Could you check a few things on this model? Use its own coordinates, in mm. A direction names the side the tool comes from. Give positions to 0.01 mm unless a question says otherwise; leave off trailing zeros. Loops run counter-clockwise (first coordinate to the right, second up) from the corner with the lowest first, then second, coordinate; pieces in that order, holes last. Notation, with made-up numbers: (44.25, -10) - (103.25, -10) arc R13 ccw to (103.25, 2) - close; hole circle Ø1 at (42.25, -5.75). An arc over 180 degrees is marked (long way). Answer in a Markdown table with one row per item. Add a question column.
```python
from build123d import *
from OCP.BRepFilletAPI import BRepFilletAPI_MakeChamfer

# Parameters (mm, degrees)
SKETCH1_W                     = 20
SKETCH1_H                     = 40.56076
BOSS_EXTRUDE1_DEPTH           = 8
SKETCH6_R                     = 1.4
CUT_EXTRUDE1_DEPTH            = 10
SKETCH8_R                     = 7.5
BOSS_EXTRUDE2_DEPTH           = 2.5
SKETCH9_R                     = 5.1
CUT_EXTRUDE3_DEPTH            = 4
SKETCH10_R                    = 3
CUT_EXTRUDE4_DEPTH            = 6.5
FILLET1_R                     = 2
CHAMFER1_SIZE2                = 2.5
CHAMFER1_SIZE                 = 1.8
SKETCH11_W                    = 8
SKETCH11_H                    = 7
CUT_EXTRUDE5_DEPTH            = 3.5
CHAMFER2_SIZE                 = 2.020725942
CHAMFER2_SIZE_2               = 3.5
FILLET2_R                     = 3
BODY_MOVE_COPY1_OUTLINE_W     = 2.1
BODY_MOVE_COPY1_OUTLINE_H     = 6.5
BODY_MOVE_COPY1_START         = -10
BODY_MOVE_COPY1_2_DEPTH       = 20
BODY_MOVE_COPY1_3_OUTLINE_R   = 1.4
BODY_MOVE_COPY1_3_DEPTH       = 4.176980959
BODY_MOVE_COPY1_4_OUTLINE_R   = 1.4
BODY_MOVE_COPY1_4_DEPTH       = 20
BODY_MOVE_COPY1_5_OUTLINE_R   = 1.4
BODY_MOVE_COPY1_5_DEPTH       = 10
BODY_MOVE_COPY1_6_OUTLINE_R   = 5.1
BODY_MOVE_COPY1_6_DEPTH       = 2.5
BODY_MOVE_COPY1_START_2       = -16
BODY_MOVE_COPY1_7_OUTLINE_R   = 3
BODY_MOVE_COPY1_7_DEPTH       = 8
BODY_MOVE_COPY1_8_OUTLINE_R   = 5.1
BODY_MOVE_COPY1_8_OUTLINE_R_2 = 3
BODY_MOVE_COPY1_8_DEPTH       = 1.5


with BuildPart() as part:
    # Sketch1 → Boss-Extrude1 (new body)
    with BuildSketch(Plane.XY):
        Rectangle(SKETCH1_W, SKETCH1_H)
    extrude(amount=-BOSS_EXTRUDE1_DEPTH)

    # Sketch6 → Cut-Extrude1 (cut)
    with BuildSketch(Plane(origin=(10, 0, 0), x_dir=(0, 0, -1), z_dir=(1, 0, 0))):
        with Locations(Location((3.3, -15.26519, 0), (0, 0, 180))):
            Circle(SKETCH6_R)
        with Locations((3.3, -5.26519)):
            Circle(SKETCH6_R)
        with Locations((3.3, 15.26519)):
            Circle(SKETCH6_R)
        with Locations(Location((3.3, 5.26519, 0), (0, 0, 180))):
            Circle(SKETCH6_R)
    extrude(amount=-CUT_EXTRUDE1_DEPTH, mode=Mode.SUBTRACT)

    # Sketch8 → Boss-Extrude2 (add)
    with BuildSketch(Plane.XY):
        Circle(SKETCH8_R)
    extrude(amount=BOSS_EXTRUDE2_DEPTH)

    # Sketch9 → Cut-Extrude3 (cut)
    with BuildSketch(Plane.XY.offset(2.5)):
        Circle(SKETCH9_R)
    extrude(amount=-CUT_EXTRUDE3_DEPTH, mode=Mode.SUBTRACT)

    # Sketch10 → Cut-Extrude4 (cut)
    with BuildSketch(Plane.XY.offset(-1.5)):
        Circle(SKETCH10_R)
    extrude(amount=-CUT_EXTRUDE4_DEPTH, mode=Mode.SUBTRACT)

    # Fillet1
    fillet1_edges = [part.edges().sort_by_distance(p)[0] for p in [
        (0, -20.28038, 0),
        (0, 20.28038, 0),
    ]]
    fillet(fillet1_edges, radius=FILLET1_R)

    # Chamfer1
    chamfer1_edges = [part.edges().sort_by_distance(p)[0] for p in [
        (-7.5, 0, 0),
    ]]
    chamfer1_side = [part.faces().sort_by_distance(p)[0] for p in [
        (-7.536, 0, 0),
    ]]
    chamfer(chamfer1_edges, length=CHAMFER1_SIZE - 0.0001, length2=CHAMFER1_SIZE2 - 0.0001, reference=chamfer1_side[0])  # a hair under: the kernel refuses the full size

    # Sketch11 → Cut-Extrude5 (cut)
    with BuildSketch(Plane.ZY.offset(10)):
        with Locations((-4, -10.26517)):
            Rectangle(SKETCH11_W, SKETCH11_H)
    extrude(amount=-CUT_EXTRUDE5_DEPTH, mode=Mode.SUBTRACT)

    # Chamfer2
    chamfer2_edges_1 = [part.edges().sort_by_distance(p)[0] for p in [
        (-10, -13.76517, -4),
    ]]
    chamfer2_side_1 = [part.faces().sort_by_distance(p)[0] for p in [
        (-10, -13.805584519, -4),
    ]]
    chamfer2_edges_2 = [part.edges().sort_by_distance(p)[0] for p in [
        (-10, -6.76517, -4),
    ]]
    chamfer2_side_2 = [part.faces().sort_by_distance(p)[0] for p in [
        (-9.959585481, -6.76517, -4),
    ]]
    chamfer2 = BRepFilletAPI_MakeChamfer(part.part.solid().wrapped)
    for e in chamfer2_edges_1:
        chamfer2.Add(CHAMFER2_SIZE - 0.0001, CHAMFER2_SIZE_2 - 0.0001, e.wrapped, chamfer2_side_1[0].wrapped)
    for e in chamfer2_edges_2:
        chamfer2.Add(CHAMFER2_SIZE_2 - 0.0001, CHAMFER2_SIZE - 0.0001, e.wrapped, chamfer2_side_2[0].wrapped)
    add(Compound.cast(chamfer2.Shape()), mode=Mode.REPLACE)  # a hair under: the kernel refuses the full size

    # Fillet2
    fillet2_edges = [part.edges().sort_by_distance(p)[0] for p in [
        (-10, -15.785795942, -4),
        (-10, -4.744544058, -4),
    ]]
    fillet(fillet2_edges, radius=FILLET2_R)

    # Body-Move/Copy1: read off the stored shape, not the designer's step
    # Body-Move/Copy1 outline → Body-Move/Copy1 (revolve)
    with BuildSketch(Plane.XZ):
        Polygon((7.5, -18.5), (9.3, -16), (5.1, -16), (5.1, -18.5), align=None)
        with Locations((4.05, -11.25)):
            Rectangle(BODY_MOVE_COPY1_OUTLINE_W, BODY_MOVE_COPY1_OUTLINE_H)
    revolve(axis=Axis((0, 0, 0), (0, 0, 1)))

    # Body-Move_Copy1 2 outline → Body-Move_Copy1 2 (cut)
    with BuildSketch(Plane.YZ.offset(BODY_MOVE_COPY1_START)):
        with BuildLine():
            Line((-20.28038, -8), (20.28038, -8))
            Line((20.28038, -8), (20.28038, -2))
            ThreePointArc((20.28038, -2), (19.694593562, -0.585786438), (18.28038, 0))
            Line((18.28038, 0), (-18.28038, 0))
            ThreePointArc((-18.28038, 0), (-19.694593562, -0.585786438), (-20.28038, -2))
            Line((-20.28038, -2), (-20.28038, -8))
        make_face()
    extrude(amount=BODY_MOVE_COPY1_2_DEPTH, mode=Mode.SUBTRACT)

    # Body-Move_Copy1 3 outline → Body-Move_Copy1 3 (cut)
    with BuildSketch(Plane.YZ):
        with Locations((-5.26519, -12.7)):
            Circle(BODY_MOVE_COPY1_3_OUTLINE_R)
        with Locations((5.26519, -12.7)):
            Circle(BODY_MOVE_COPY1_3_OUTLINE_R)
    extrude(amount=BODY_MOVE_COPY1_3_DEPTH, mode=Mode.SUBTRACT)

    # Body-Move_Copy1 4 outline → Body-Move_Copy1 4 (add)
    with BuildSketch(Plane.YZ.offset(BODY_MOVE_COPY1_START)):
        with BuildLine():
            ThreePointArc((18.28038, -16), (19.694593562, -15.414213562), (20.28038, -14))
            Line((20.28038, -14), (20.28038, -8))
            Line((20.28038, -8), (-20.28038, -8))
            Line((-20.28038, -8), (-20.28038, -14))
            ThreePointArc((-20.28038, -14), (-19.694593562, -15.414213562), (-18.28038, -16))
            Line((-18.28038, -16), (18.28038, -16))
        make_face()
        with Locations((-15.26519, -12.7)):
            Circle(BODY_MOVE_COPY1_4_OUTLINE_R, mode=Mode.SUBTRACT)
        with Locations((-5.26519, -12.7)):
            Circle(BODY_MOVE_COPY1_4_OUTLINE_R, mode=Mode.SUBTRACT)
        with Locations((5.26519, -12.7)):
            Circle(BODY_MOVE_COPY1_4_OUTLINE_R, mode=Mode.SUBTRACT)
        with Locations((15.26519, -12.7)):
            Circle(BODY_MOVE_COPY1_4_OUTLINE_R, mode=Mode.SUBTRACT)
    extrude(amount=BODY_MOVE_COPY1_4_DEPTH)

    # Body-Move_Copy1 5 outline → Body-Move_Copy1 5 (add)
    with BuildSketch(Plane.YZ.offset(BODY_MOVE_COPY1_START)):
        with Locations((-5.26519, -12.7)):
            Circle(BODY_MOVE_COPY1_5_OUTLINE_R)
        with Locations((15.26519, -12.7)):
            Circle(BODY_MOVE_COPY1_5_OUTLINE_R)
        with Locations((5.26519, -12.7)):
            Circle(BODY_MOVE_COPY1_5_OUTLINE_R)
        with Locations((-15.26519, -12.7)):
            Circle(BODY_MOVE_COPY1_5_OUTLINE_R)
    extrude(amount=BODY_MOVE_COPY1_5_DEPTH)

    # Body-Move_Copy1 6 outline → Body-Move_Copy1 6 (cut)
    with BuildSketch(Plane.XY):
        with BuildLine():
            Line((-6.5, -6.76517), (-6.5, -13.76517))
            Line((-6.5, -13.76517), (-8.5, -14.919870538))
            ThreePointArc((-8.5, -14.919870538), (-9.598076211, -16.01794675), (-10, -17.51794675))
            Line((-10, -17.51794675), (-10, -19))
            Line((-10, -19), (11, -19))
            Line((11, -19), (11, 11))
            Line((11, 11), (-10.000000008, 11))
            Line((-10.000000008, 11), (-10, -3.01239325))
            ThreePointArc((-10, -3.01239325), (-9.598076211, -4.51239325), (-8.5, -5.610469462))
            Line((-8.5, -5.610469462), (-6.5, -6.76517))
        make_face()
        Circle(BODY_MOVE_COPY1_6_OUTLINE_R, mode=Mode.SUBTRACT)
    extrude(amount=BODY_MOVE_COPY1_6_DEPTH, mode=Mode.SUBTRACT)

    # Body-Move_Copy1 7 outline → Body-Move_Copy1 7 (cut)
    with BuildSketch(Plane.XY.offset(BODY_MOVE_COPY1_START_2)):
        Circle(BODY_MOVE_COPY1_7_OUTLINE_R)
        with BuildLine():
            Line((-8.5, -14.919870538), (-6.5, -13.76517))
            Line((-6.5, -13.76517), (-6.5, -6.76517))
            Line((-6.5, -6.76517), (-8.5, -5.610469462))
            ThreePointArc((-8.5, -5.610469462), (-9.598076211, -4.51239325), (-10, -3.01239325))
            Line((-10, -3.01239325), (-10, -17.51794675))
            ThreePointArc((-10, -17.51794675), (-9.598076211, -16.01794675), (-8.5, -14.919870538))
        make_face()
    extrude(amount=BODY_MOVE_COPY1_7_DEPTH, mode=Mode.SUBTRACT)

    # Body-Move_Copy1 8 outline → Body-Move_Copy1 8 (cut)
    with BuildSketch(Plane.XY.offset(BODY_MOVE_COPY1_START_2)):
        Circle(BODY_MOVE_COPY1_8_OUTLINE_R)
        Circle(BODY_MOVE_COPY1_8_OUTLINE_R_2, mode=Mode.SUBTRACT)
    extrude(amount=BODY_MOVE_COPY1_8_DEPTH, mode=Mode.SUBTRACT)


solid = part.part
```
(1) On a 3-axis mill with a long thin cutter (end or side, diameter ignored), from which of +Z, -Z, +X, -X, +Y, -Y can I reach the whole of each face in a straight line? I mean faces 4 (the cylindrical face through (-9.59, -4.53, -12.06)), 5 (the flat face through (3.3, 0.1, -14.5)), 6 (the flat face through (0, 15, -13)). Say none if no direction works.
(2) I want a section at C-C on z = -12.7. Please give me the cut outline in (x, y).
(3) For pin 1 Ø1.4 at (y, z) = (-5, -12.5) entering from +X; pin 2 Ø12 at (x, y) = (-3, 15.5) entering from -Z; pin 3 Ø1.5 at (x, y) = (2.5, 3) entering from -Z; pin 4 Ø3.5 at (x, y) = (0, 0) entering from -Z, each with a flat end and sliding along its axis, tell me the tip position at first contact or that it passes through.
(4) I want a section at D-D on y = -16. Please give me the cut outline in (x, z).
(5) Please list where these lines run through material, in increasing order: line 1 (Z direction, x = 3, y = 15.5); line 2 (Z direction, x = 5.5, y = 11); line 3 (Y direction, x = 0, z = -10.5).
(6) I want a section at A-A on z = -9. Please give me the cut outline in (x, y), then the cut area to 3 significant figures.
(7) I want a section at B-B on y = 0. Please give me the cut outline in (x, z).
(8) We'd pull the mould along Z, two halves only. Please class faces 1 (the cylindrical face through (4.93, 14.962, -14.067)), 2 (the flat face through (-10, -19, -12)), 3 (the flat face through (9, 4, -16)): pulls with the +Z half, pulls with the -Z half, needs draft (parallel to the pull), parting line crosses it, or undercut.
Reported:
| question | item | result |
|---|---|---|
| 1 | face 4 | +Z, -Z, -X |
| 1 | face 5 | -Z |
| 1 | face 6 | +X |
| 2 | outline | (-10, -20.28) - (10, -20.28) - (10, -16.67) - (0, -16.67) - (0, -13.87) - (10, -13.87) - (10, -6.67) - (0, -6.67) - (0, -3.87) - (10, -3.87) - (10, 3.87) - (0, 3.87) - (0, 6.67) - (10, 6.67) - (10, 13.87) - (0, 13.87) - (0, 16.67) - (10, 16.67) - (10, 20.28) - (-10, 20.28) - (-10, -3.01) arc R3 ccw to (-8.5, -5.61) - (-6.5, -6.77) - (-6.5, -13.77) - (-8.5, -14.92) arc R3 ccw to (-10, -17.52) - close; hole circle Ø6 at (0, 0) |
| 3 | pin 1 | x = 0 |
| 3 | pin 2 | z = -16 |
| 3 | pin 3 | z = -14.5 |
| 3 | pin 4 | through |
| 4 | outline | (-9.59, -16) - (10, -16) - (10, -13.89) - (0, -13.89) - (0, -11.51) - (10, -11.51) - (10, -8) - (-9.59, -8) - close |
| 5 | line 1 | -16 to -14.08, -11.32 to -8 |
| 5 | line 2 | -16 to -8 |
| 5 | line 3 | -20.28 to -3, 3 to 20.28 |
| 6 | outline | (-10, -20.28) - (10, -20.28) - (10, 20.28) - (-10, 20.28) - (-10, -3.01) arc R3 ccw to (-8.5, -5.61) - (-6.5, -6.77) - (-6.5, -13.77) - (-8.5, -14.92) arc R3 ccw to (-10, -17.52) - close; hole circle Ø6 at (0, 0) |
| 6 | area | 750 mm² |
| 7 | outline | (-10, -16) - (-9.3, -16) - (-7.5, -18.5) - (-5.1, -18.5) - (-5.1, -14.5) - (-3, -14.5) - (-3, -8) - (-10, -8) - close; (3, -14.5) - (5.1, -14.5) - (5.1, -18.5) - (7.5, -18.5) - (9.3, -16) - (10, -16) - (10, -8) - (3, -8) - close |
| 8 | face 1 | undercut |
| 8 | face 2 | needs draft |
| 8 | face 3 | pulls with the -Z half |
